```python
from build123d import *
from build123d.topology import SkipClean

# Parameters (mm, degrees)
BOSS_EXTRUDE1_DEPTH = 2
SKETCH2_W           = 25
SKETCH2_H           = 2
BOSS_EXTRUDE2_DEPTH = 10
SKETCH3_R           = 1.6
CUT_EXTRUDE1_DEPTH  = 10
FILLET5_START       = -12.5
FILLET5_DEPTH       = 25
FILLET5_2_DEPTH     = 4
FILLET5_START_2     = 8.5
FILLET5_3_DEPTH     = 4
FILLET5_4_OUTLINE_R = 1.6
FILLET5_4_DEPTH     = 3.35
CUT_EXTRUDE3_DEPTH  = 10
BOSS_EXTRUDE3_DEPTH = 4
BOSS_EXTRUDE4_START = -21
BOSS_EXTRUDE4_DEPTH = 4
BOSS_EXTRUDE5_REACH = 25.867
SKETCH9_R           = 1.6
CUT_EXTRUDE5_DEPTH  = 10
CUT_EXTRUDE4_START  = 2
CUT_EXTRUDE4_DEPTH  = 10


with BuildPart() as part:
    # Sketch1 → Boss-Extrude1 (new body)
    with BuildSketch(Plane.XY):
        Polygon((8.5, -5.35), (12.5, -5.35), (12.5, 5.35), (-12.5, 5.35), (-12.5, -5.35), (-8.5, -5.35), (-8.5, -2.35), (8.5, -2.35), align=None)
    extrude(amount=BOSS_EXTRUDE1_DEPTH)

    # Sketch2 → Boss-Extrude2 (add)
    with BuildSketch(Plane(origin=(0, 0, 0), x_dir=(-1, 0, 0), z_dir=(0, 0, -1))):
        with Locations((0, 4.35)):
            Rectangle(SKETCH2_W, SKETCH2_H)
    extrude(amount=BOSS_EXTRUDE2_DEPTH)

    # Sketch3 → Cut-Extrude1 (cut)
    with BuildSketch(Plane(origin=(0, 5.35, 0), x_dir=(1, 0, 0), z_dir=(0, 1, 0))):
        with Locations(Location((-7, 5, 0), (0, 0, 270))):
            Circle(SKETCH3_R)
        with Locations(Location((7, 5, 0), (0, 0, 270))):
            Circle(SKETCH3_R)
    extrude(amount=-CUT_EXTRUDE1_DEPTH, mode=Mode.SUBTRACT)

    # Fillet5: read off the stored shape, not the designer's step
    # Fillet5 outline → Fillet5 (add)
    with BuildSketch(Plane.YZ.offset(FILLET5_START)):
        with BuildLine():
            Line((-2.35, 0), (-2.35, -0.886851064))
            ThreePointArc((-2.35, -0.886851064), (1.805767263, -4.576600812), (3.35, -9.915139938))
            Line((3.35, -9.915139938), (3.35, 0))
            Line((3.35, 0), (-2.35, 0))
        make_face()
    extrude(amount=FILLET5_DEPTH)

    # Fillet5 2 outline → Fillet5 2 (add)
    with BuildSketch(Plane.YZ.offset(FILLET5_START)):
        with BuildLine():
            ThreePointArc((-5.35, 0), (-3.81510561, -0.325386355), (-2.35, -0.886851064))
            Line((-2.35, -0.886851064), (-2.35, 0))
            Line((-2.35, 0), (-5.35, 0))
        make_face()
    extrude(amount=FILLET5_2_DEPTH)

    # Fillet5 3 outline → Fillet5 3 (add)
    with BuildSketch(Plane.YZ.offset(FILLET5_START_2)):
        with BuildLine():
            ThreePointArc((-5.35, 0), (-3.81510561, -0.325386355), (-2.35, -0.886851064))
            Line((-2.35, -0.886851064), (-2.35, 0))
            Line((-2.35, 0), (-5.35, 0))
        make_face()
    extrude(amount=FILLET5_3_DEPTH)

    # Fillet5 4 outline → Fillet5 4 (cut)
    with SkipClean():  # the faces are left unmerged after this step: merging them gives an invalid solid
        with BuildSketch(Plane(origin=(0, 0, 0), x_dir=(1, 0, 0), z_dir=(0, 1, 0))):
            with Locations((7, 5)):
                Circle(FILLET5_4_OUTLINE_R)
            with Locations((-7, 5)):
                Circle(FILLET5_4_OUTLINE_R)
        extrude(amount=FILLET5_4_DEPTH, mode=Mode.SUBTRACT)

    # Sketch4 → Cut-Extrude3 (cut)
    with BuildSketch(Plane(origin=(0, 3.35, 0), x_dir=(1, 0, 0), z_dir=(0, 1, 0))):
        Polygon((-3.709103466, 5), (-5.354551733, 7.85), (-8.645448267, 7.85), (-10.290896534, 5), (-8.645448267, 2.15), (-5.354551733, 2.15), align=None)
        Polygon((3.709103466, 5), (5.354551733, 2.15), (8.645448267, 2.15), (10.290896534, 5), (8.645448267, 7.85), (5.354551733, 7.85), align=None)
    extrude(amount=-CUT_EXTRUDE3_DEPTH, mode=Mode.SUBTRACT)

    # Sketch7 → Boss-Extrude3 (add)
    with BuildSketch(Plane.ZY.offset(12.5)):
        Polygon((2, -5.35), (2.9361287, -5.35), (2, 5.35), align=None)
    extrude(amount=-BOSS_EXTRUDE3_DEPTH)

    # Sketch7<2> → Boss-Extrude4 (add)
    with BuildSketch(Plane.ZY.offset(12.5).offset(BOSS_EXTRUDE4_START)):
        Polygon((2, -5.35), (2.9361287, -5.35), (2, 5.35), align=None)
    extrude(amount=-BOSS_EXTRUDE4_DEPTH)

    # Sketch10 → Boss-Extrude5 (add, up to next)
    with BuildSketch(Plane.ZY.offset(-8.5), mode=Mode.PRIVATE) as boss_extrude5_sk1:
        Polygon((2, -2.35), (2.673662709, -2.35), (2, 5.35), align=None)
    boss_extrude5_tool1 = extrude(boss_extrude5_sk1.sketch, amount=BOSS_EXTRUDE5_REACH, mode=Mode.PRIVATE) - part.part
    add(boss_extrude5_tool1.solids().sort_by_distance((8.5, 0.216667, 2.224554))[0])

    # Sketch9 → Cut-Extrude5 (cut)
    with BuildSketch(Plane(origin=(0, 0.214287438, 2.449316628), x_dir=(1, 0, 0), z_dir=(0, 0.08715574274766177, 0.9961946980917453))):
        with Locations(Location((-10, 0, 0), (0, 0, 270))):
            Circle(SKETCH9_R)
        with Locations(Location((10, 0, 0), (0, 0, 270))):
            Circle(SKETCH9_R)
    extrude(amount=-CUT_EXTRUDE5_DEPTH, mode=Mode.SUBTRACT)

    # Sketch6 → Cut-Extrude4 (cut)
    with BuildSketch(Plane(origin=(0, 10.679641635, 1.533716776), x_dir=(1, 0, 0), z_dir=(0, -0.08715574274766179, -0.9961946980917453)).offset(CUT_EXTRUDE4_START)):
        Polygon((-6.709103466, 10.505330149), (-8.354551733, 13.355330149), (-11.645448267, 13.355330149), (-13.290896534, 10.505330149), (-11.645448267, 7.655330149), (-8.354551733, 7.655330149), align=None)
        Polygon((6.709103466, 10.505330149), (8.354551733, 7.655330149), (11.645448267, 7.655330149), (13.290896534, 10.505330149), (11.645448267, 13.355330149), (8.354551733, 13.355330149), align=None)
    extrude(amount=CUT_EXTRUDE4_DEPTH, mode=Mode.SUBTRACT)


solid = part.part
```
Geometry: final body of the model. Coordinates: model frame, mm. A direction names the side the tool comes from. Round coordinates to 2 decimals unless told otherwise and drop trailing zeros. Loops run counter-clockwise (first coordinate to the right, second up) from the corner with the lowest first, then second, coordinate; pieces in that order, holes last. Notation, with made-up numbers: (68.25, 88) -> (98.25, 88) arc R25 ccw to (98.25, 109) -> close; hole circle Ø6 at (10, 8.5). An arc over 180 degrees is marked (long way). Use one line per item in the form item = value.
Item 1: Cut plane A-A on z = -4.25. Output: boundary loops of the cut face in (x, y).
Evaluation:
outline = (-12.5, 1.59) -> (-12.16, 1.59) -> (-11.65, 2.49) -> (-9.86, 2.49) -> (-9.86, 3.35) -> (-8.41, 3.35) -> (-8.41, 5.35) -> (-12.5, 5.35) -> close; (-5.59, 3.35) -> (-4.14, 3.35) -> (-4.14, 1.59) -> (4.14, 1.59) -> (4.14, 3.35) -> (5.59, 3.35) -> (5.59, 5.35) -> (-5.59, 5.35) -> close; (8.41, 3.35) -> (9.86, 3.35) -> (9.86, 2.49) -> (11.65, 2.49) -> (12.16, 1.59) -> (12.5, 1.59) -> (12.5, 5.35) -> (8.41, 5.35) -> close
Item 2: Cut plane D-D on z = -9. Output: boundary loops of the cut face in (x, y), then the cut area to 3 significant figures.
Evaluation:
outline = (-12.5, 3.31) -> (12.5, 3.31) -> (12.5, 5.35) -> (-12.5, 5.35) -> close
area = 51.0 mm2
Item 3: Cut plane C-C on x = 2.25. Output: boundary loops of the cut face in (y, z), then the cut area to 3 significant figures.
Evaluation:
outline = (-2.35, -0.89) arc R10 cw to (3.35, -9.92) -> (3.35, -10) -> (5.35, -10) -> (5.35, 2) -> (-2.35, 2.67) -> close
area = 57.6 mm2
Item 4: Access query for faces 4 (the flat face through (-10.389, 2.685, -2.01)), 5 (the flat face through (-10.051, -2.857, 0.043)), 6 (the flat face through (4.7, 1.94, -3.28)), 7 (the flat face through (0, -2.35, 1)). Directions: +Z, -Z, +X, -X, +Y, -Y. A direction counts if a zero-diameter tool reaches every point of the face in a straight line with its end or side. Return the directions, or none.
Evaluation:
face_4 = none
face_5 = -Z
face_6 = -Y
face_7 = +Z, -Z, -Y
Item 5: Contact query for flat-ended pins moving along their axis: pin 1 Ø2.5 at (x, y) = (7, 1.5) entering from -Z; pin 2 Ø4 at (x, z) = (7, -5) entering from -Y; pin 3 Ø4 at (x, z) = (0, 1) entering from -Y; pin 4 Ø2 at (y, z) = (0.5, -5.5) entering from +X. Output: stop coordinate, or through.
Evaluation:
pin_1 = -2.15
pin_2 = 3.35
pin_3 = -2.35
pin_4 = through
Item 6: Material intervals for probe 1 along X at (y, z) = (4.15, -5); probe 2 along X at (y, z) = (0, 2); probe 3 along Z at (x, y) = (10, 4.75), sorted ascending.
Evaluation:
probe_1 = -12.5 to -8.6, -5.4 to 5.4, 8.6 to 12.5
probe_2 = -12.5 to -11.59, -8.41 to 8.41, 11.59 to 12.5
probe_3 = -10 to 2.05
Item 7: Cut plane B-B on y = -3.5. Output: boundary loops of the cut face in (x, z), then the cut area to 3 significant figures.
Evaluation:
outline = (-12.5, -0.42) -> (-8.5, -0.42) -> (-8.5, 2.77) -> (-12.5, 2.77) -> close; (8.5, -0.42) -> (12.5, -0.42) -> (12.5, 2.77) -> (8.5, 2.77) -> close
area = 25.6 mm2
Item 8: Draft query along Y for faces 1 (the flat face through (10, -5.35, 1)), 2 (the flat face through (-7, 2, -2.15)), 3 (the flat face through (-7.392, -1.226, -0.441)). Return one class per face: released by +Y, released by -Y, zero draft, split by the parting line, or undercut.
Evaluation:
face_1 = released by -Y
face_2 = zero draft
face_3 = undercut
